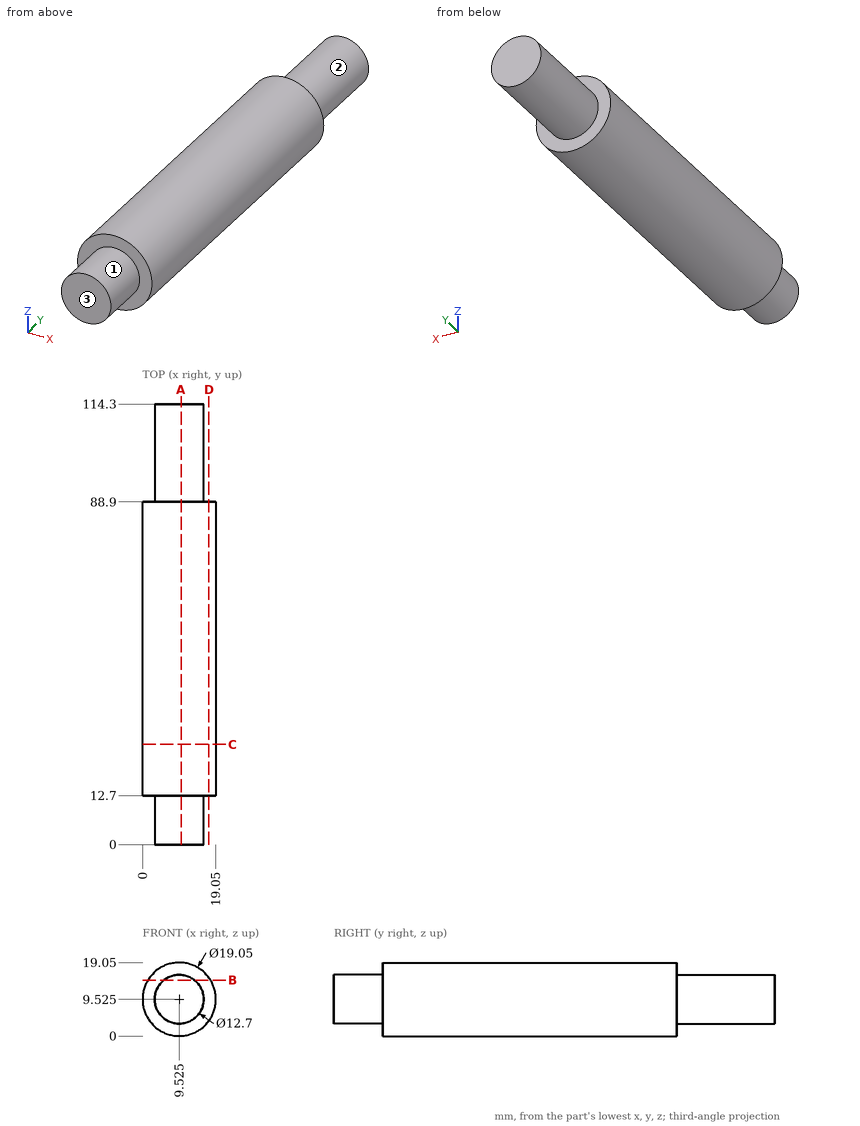
For this review, use the dimensioned drawing (mm, ordinates from the lowest corner) and the shaded views. A direction names the side the tool comes from. Round coordinates to 2 decimals unless told otherwise and drop trailing zeros. Write each loop counter-clockwise with the first axis right and the second up, starting at its lowest first coordinate (ties: lowest second). Pieces come first, ordered by that corner, then holes. Notation, with made-up numbers: (43.25, 52.5) -> (50.25, 52.5) arc R13 cw to (50.25, 75.5) -> close; hole circle Ø9 at (26, 57.5). An arc over 180 degrees is marked (long way). One line per item, written item: value. Start each with the question number.
Q1. Add section A-A (x = 10). Give the boundary of the cut face in (y, z), then the cut area to 3 significant figures.
Q2. To check wall thickness, follow probe 1 along Z at (x, y) = (9, 81.5); probe 2 along Y at (x, z) = (15, 4); probe 3 along X at (y, z) = (42, 9.75). State the ranges of each line that lie inside material, in increasing order.
Q3. Insertion check: P1, Ø3, axis at x = 11.5, y = 94.5, coming from the -Z side; P2, Ø3, axis at x = 8.5, y = 94, coming from the +Z side (3 decimals); P3, Ø1, axis at x = 3.5, z = 15.5, coming from the -Y side. Each pin has a flat end and moves straight along its axis. Give the tip position at first contact, or say it passes through.
Q4. Add section B-B (z = 14.5). Give the boundary of the cut face in (x, y).
Q5. Tool access review of the marked faces 1, 2 and 3: name each direction out of +Z, -Z, +X, -X, +Y, -Y from which nothing blocks a thin tool from reaching the whole face with its end or side.
Q6. Add section D-D (x = 17.25). Give the boundary of the cut face in (y, z).
Q7. Add section C-C (y = 26). Give the boundary of the cut face in (x, z) (3 decimals), then the cut area to 3 significant figures.
Response:
1. outline: (0, 3.19) -> (12.7, 3.19) -> (12.7, 0.01) -> (88.9, 0.01) -> (88.9, 3.19) -> (114.3, 3.19) -> (114.3, 15.86) -> (88.9, 15.86) -> (88.9, 19.04) -> (12.7, 19.04) -> (12.7, 15.86) -> (0, 15.86) -> close
1. area: 1,930 mm^2
2. probe 1: z = 0.01 to 19.04
2. probe 2: y = 12.7 to 88.9
2. probe 3: x = 0 to 19.05
3. P1: stops at z = 3.19
3. P2: stops at z = 15.875
3. P3: stops at y = 12.7
4. outline: (1.4, 12.7) -> (5.58, 12.7) -> (5.58, 0) -> (13.47, 0) -> (13.47, 12.7) -> (17.65, 12.7) -> (17.65, 88.9) -> (13.47, 88.9) -> (13.47, 114.3) -> (5.58, 114.3) -> (5.58, 88.9) -> (1.4, 88.9) -> close
5. face 1: -Y
5. face 2: +Y
5. face 3: +Z, -Z, +X, -X, -Y
6. outline: (12.7, 3.95) -> (88.9, 3.95) -> (88.9, 15.1) -> (12.7, 15.1) -> close
7. outline: circle Ø19.05 at (9.525, 9.525)
7. area: 285 mm^2
